from build123d import *

# Parameters (mm, degrees)
F1_DEPTH = 11
F3_DEPTH = 5
F4_R     = 12
F4_R_2   = 19.649639
F5_DEPTH = 11
F7_DEPTH = 16
F8_W     = 9
F8_H     = 5
F9_DEPTH = 136.650639


with BuildPart() as f1:
    # F0 (on Top) → F1 (new body)
    with BuildSketch(Plane.XY):
        with BuildLine():
            Line((-16, 76), (-59, 76))
            ThreePointArc((-59, 76), (-73.632156, 66.473021), (-70.839282, 49.237501))
            Line((-70.839282, 49.237501), (-34.640628, 9.417187))
            ThreePointArc((-34.640628, 9.417187), (-31.941838, 5.048207), (-31, 0))
            ThreePointArc((-31, 0), (-31.941838, -5.048207), (-34.640628, -9.417187))
            Line((-34.640628, -9.417187), (-70.839282, -49.237501))
            ThreePointArc((-70.839282, -49.237501), (-73.632156, -66.473021), (-59, -76))
            Line((-59, -76), (-16, -76))
            ThreePointArc((-16, -76), (-4.686292, -71.313708), (0, -60))
            Line((0, -60), (0, 0))
            Line((0, 0), (0, 60))
            ThreePointArc((0, 60), (-4.686292, 71.313708), (-16, 76))
        make_face()
        with BuildLine():
            Line((-59, -50), (-16, -50))
            ThreePointArc((-16, -50), (-6, -60), (-16, -70))
            Line((-16, -70), (-59, -70))
            ThreePointArc((-59, -70), (-69, -60), (-59, -50))
        make_face(mode=Mode.SUBTRACT)
        with BuildLine():
            ThreePointArc((-59, 50), (-69, 60), (-59, 70))
            Line((-59, 70), (-16, 70))
            ThreePointArc((-16, 70), (-6, 60), (-16, 50))
            Line((-16, 50), (-59, 50))
        make_face(mode=Mode.SUBTRACT)
    extrude(amount=F1_DEPTH)

    # F2 (on face) → F3 (join)
    with BuildSketch(Plane.XY.offset(11)):
        with BuildLine():
            ThreePointArc((-50.206183, 34), (-52.949713, 32.213692), (-52.426049, 28.982031))
            Line((-52.426049, 28.982031), (-34.640628, 9.417187))
            ThreePointArc((-34.640628, 9.417187), (-31, 0), (-34.640628, -9.417187))
            Line((-34.640628, -9.417187), (-52.426049, -28.982031))
            ThreePointArc((-52.426049, -28.982031), (-52.949713, -32.213692), (-50.206183, -34))
            Line((-50.206183, -34), (0, -34))
            Line((0, -34), (0, 34))
            Line((0, 34), (-50.206183, 34))
        make_face()
    extrude(amount=F3_DEPTH)

    # F4 (on Front) → F5 (join, symmetric)
    with BuildSketch(Plane.XZ):
        with BuildLine():
            Line((0, 16), (0, 0))
            Line((0, 0), (35, 0))
            ThreePointArc((35, 0), (39.242641, -1.757359), (41, -6))
            Line((41, -6), (41, -38))
            ThreePointArc((41, -38), (42.757359, -42.242641), (47, -44))
            Line((47, -44), (97, -44))
            ThreePointArc((97, -44), (101.242641, -42.242641), (103, -38))
            Line((103, -38), (103, -5.649639))
            ThreePointArc((103, -5.649639), (104.757359, -1.406998), (109, 0.350361))
            ThreePointArc((109, 0.350361), (134.983932, 37.451867), (91.23509, 49.187508))
            ThreePointArc((91.23509, 49.187508), (48.541869, 24.554554), (0, 16))
        make_face()
        with Locations((72, -26)):
            Circle(F4_R, mode=Mode.SUBTRACT)
        with Locations((109, 28)):
            Circle(F4_R_2, mode=Mode.SUBTRACT)
    extrude(amount=F5_DEPTH, both=True)

    # F6 (on Top) → F7 (join, through all)
    with BuildSketch(Plane.XY):
        with BuildLine():
            ThreePointArc((32, 11), (9.372583, 20.372583), (0, 43))
            Line((0, 43), (0, 34))
            Line((0, 34), (0, 11))
            Line((0, 11), (32, 11))
        make_face()
        with BuildLine():
            Line((0, -34), (0, -43))
            ThreePointArc((0, -43), (9.372583, -20.372583), (32, -11))
            Line((32, -11), (0, -11))
            Line((0, -11), (0, -34))
        make_face()
    extrude(amount=F7_DEPTH)

    # F8 (on Right) → F9 (cut, through all)
    with BuildSketch(Plane.YZ):
        with Locations((38.5, 13.5)):
            Rectangle(F8_W, F8_H)
        with Locations((-38.5, 13.5)):
            Rectangle(F8_W, F8_H)
    extrude(amount=F9_DEPTH, mode=Mode.SUBTRACT)


solid = f1.part
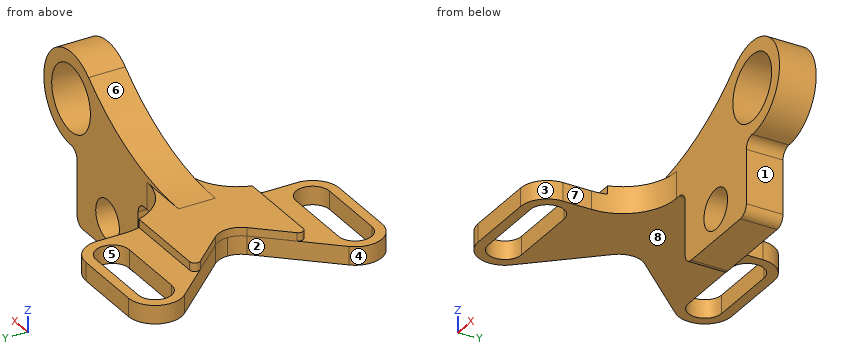
Geometry: final body of the model. Coordinates: model frame, mm. Face numbers are marked on the shaded views. A direction names the side the tool comes from. Coordinates: 2 decimals unless noted, no trailing zeros. Order: outer loops, then holes, each group sorted by start corner. A loop starts at its lowest first (then second) coordinate and runs counter-clockwise, first axis right, second up. Notation, with made-up numbers: (36.25, -24.5) - (84.25, -24.5) arc R23 cw to (84.25, -12.5) - close; hole circle Ø3 at (-6, 31). An arc over 180 degrees is marked (long way). Use one line per item in the form item = value.
1) Set-up query: the marked faces 4, 5, 6, 7 and 8. Return all of +Z, -Z, +X, -X, +Y, -Y with unobstructed straight access to the full face (end or side cutting, diameter ignored); none if empty.
Solutions:
face_4 = +Z, -Z, -X
face_5 = +Z, -Z
face_6 = +Z, -X, +Y, -Y
face_7 = +Z, -Z, +X, -Y
face_8 = -Z, -X, +Y, -Y
2) Ray query, L1, parallel to Z at x = 109, y = 4; L2, parallel to Y at x = 102, z = -27; L3, parallel to Z at x = -50, y = 46.5. Return the intervals inside material, ascending.
Solutions:
L1 = 0.35 to 8.35, 47.65 to 55.65
L2 = -11 to 11
L3 = 0 to 11
3) Mould query, pull axis Y, two halves, no side actions, for the marked faces 1, 2 and 3. Classes: +Y half, -Y half, draft (parallel to the pull), parting line (faces both ways), or undercut.
Solutions:
face_1 = draft
face_2 = undercut
face_3 = -Y half
4) Section C-C (y = -47). Return loops of the section in (x, z), then the cut area to 3 significant figures.
Solutions:
outline = (-68.81, 0) - (0, 0) - (0, 11) - (-68.81, 11) - close
area = 757 mm^2
5) Section A-A (x = 70). Return loops of the section in (y, z), then the cut area to 3 significant figures.
Solutions:
outline = (-11, -44) - (11, -44) - (11, -37.83) - (-11, -37.83) - close; (-11, -14.17) - (11, -14.17) - (11, 34.45) - (-11, 34.45) - close
area = 1,210 mm^2
6) Pin query (flat end, axial travel): pin 1 (9 mm diameter, centred on y = -51, z = 6.5, fed in from +X); pin 2 (6 mm diameter, centred on x = -28.5, y = 46.5, fed in from -Z); pin 3 (3 mm diameter, centred on y = 0, z = 44, fed in from +X). Return the tip coordinate at first contact, or that it passes through.
Solutions:
pin_1 = 0
pin_2 = 0
pin_3 = 132.54
7) Section B-B (z = -33). Return loops of the section in (x, y), then the cut area to 3 significant figures.
Solutions:
outline = (41, -11) - (62.25, -11) - (62.25, 11) - (41, 11) - close; (81.75, -11) - (103, -11) - (103, 11) - (81.75, 11) - close
area = 935 mm^2
